Read the model definition and answer for the solid it produces. Units are mm, in the model's axes. Face numbers are marked on the shaded views. A direction names the side the tool comes from. Give positions to 0.01 mm unless a question says otherwise; leave off trailing zeros. Write each loop counter-clockwise with the first axis right and the second up, starting at its lowest first coordinate (ties: lowest second). Pieces come first, ordered by that corner, then holes.
```python
from build123d import *

# Parameters (mm, degrees)
SKETCH1_W           = 19.05
SKETCH1_H           = 57.15
BOSS_EXTRUDE1_DEPTH = 25.4
SKETCH2_W           = 17.4625
SKETCH2_H           = 19.05
SKETCH2_W_2         = 9.525
CUT_EXTRUDE1_DEPTH  = 20.05
SKETCH9_R           = 3.175
CUT_EXTRUDE3_DEPTH  = 40.6875
FILLET1_R           = 6.35
HOLE1_D             = 7.874
CHAMFER1_SIZE       = 0.508


with BuildPart() as part:
    # Sketch1 → Boss-Extrude1 (new body)
    with BuildSketch(Plane(origin=(0, 0, 0), x_dir=(1, 0, 0), z_dir=(0, 1, 0))):
        with Locations((69.85, 0)):
            Rectangle(SKETCH1_W, SKETCH1_H)
    extrude(amount=BOSS_EXTRUDE1_DEPTH)

    # Sketch2 → Cut-Extrude1 (cut, through all)
    with BuildSketch(Plane(origin=(79.375, 0, 0), x_dir=(0, 0, -1), z_dir=(1, 0, 0))):
        with Locations((-19.84375, 15.875)):
            Rectangle(SKETCH2_W, SKETCH2_H)
        with Locations((0, 15.875)):
            Rectangle(SKETCH2_W_2, SKETCH2_H)
        with Locations((19.84375, 15.875)):
            Rectangle(SKETCH2_W, SKETCH2_H)
    extrude(amount=-CUT_EXTRUDE1_DEPTH, mode=Mode.SUBTRACT)

    # Sketch9 → Cut-Extrude3 (cut, through all)
    with BuildSketch(Plane.XY.offset(11.1125)):
        with Locations((69.85, 19.05)):
            Circle(SKETCH9_R)
    extrude(amount=-CUT_EXTRUDE3_DEPTH, mode=Mode.SUBTRACT)

    # Fillet1
    fillet1_edges = [part.edges().sort_by_distance(p)[0] for p in [
        (79.375, 25.4, 7.9375),
        (79.375, 3.175, 28.575),
        (60.325, 3.175, 28.575),
        (79.375, 25.4, -7.9375),
        (60.325, 25.4, -7.9375),
        (60.325, 25.4, 7.9375),
        (60.325, 3.175, -28.575),
        (79.375, 3.175, -28.575),
    ]]
    fillet(fillet1_edges, radius=FILLET1_R)

    # Hole1 (through all)
    with Locations(Plane(origin=(0, 6.35, 0), x_dir=(1, 0, 0), z_dir=(0, 1, 0))):
        with Locations((69.923370565, 18.735910675), (69.923370565, -18.735910675)):
            Hole(HOLE1_D / 2)

    # Chamfer1
    chamfer1_edges = [part.edges().sort_by_distance(p)[0] for p in [
        (73.860370565, 6.35, 18.735910675),
        (73.860370565, 0, 18.735910675),
        (73.860370565, 6.35, -18.735910675),
        (73.860370565, 0, -18.735910675),
    ]]
    chamfer(chamfer1_edges, length=CHAMFER1_SIZE)


solid = part.part
```
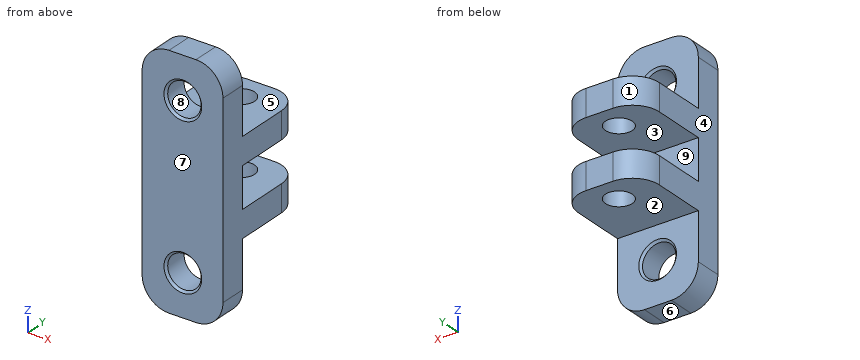
Item 1: Section C-C (y = 21.5) is taken. Write down the section's boundary in (x, z), and give its area (3 significant figures).
Result set:
outline: (60.82, -11.11) - (67.83, -11.11) - (67.83, -4.76) - (60.82, -4.76) - close; (60.82, 4.76) - (67.83, 4.76) - (67.83, 11.11) - (60.82, 11.11) - close; (71.87, -11.11) - (78.88, -11.11) - (78.88, -4.76) - (71.87, -4.76) - close; (71.87, 4.76) - (78.88, 4.76) - (78.88, 11.11) - (71.87, 11.11) - close
area: 178 mm2
Item 2: Section D-D (y = 2.25) is taken. Write down the section's boundary in (x, z) (3 decimals).
Result set:
outline: (60.325, -22.225) arc R6.35 ccw to (66.675, -28.575) - (73.025, -28.575) arc R6.35 ccw to (79.375, -22.225) - (79.375, 22.225) arc R6.35 ccw to (73.025, 28.575) - (66.675, 28.575) arc R6.35 ccw to (60.325, 22.225) - close; hole circle Ø7.874 at (69.923, -18.736); hole circle Ø7.874 at (69.923, 18.736)
Item 3: Determine the mould class of the marked faces 6, 7, 8 and 9 for opening direction Z: pulls with the +Z half, pulls with the -Z half, needs draft (parallel to the pull), parting line crosses it, or undercut.
Result set:
face 6: pulls with the -Z half
face 7: needs draft
face 8: undercut
face 9: undercut
Item 4: Which of the six approach directions +Z, -Z, +X, -X, +Y, -Y give full straight-line access (tool end or side, diameter ignored) to the marked faces 1, 2, 3, 4 and 5?
Result set:
face 1: +Z, -Z, -X, +Y
face 2: -Z, +X, -X, +Y
face 3: +X, -X, +Y
face 4: +Z, -Z, -X, +Y, -Y
face 5: +Z, +X, -X, +Y
Item 5: Each of these flat-tipped pins is pushed along its axis until it touches: pin 1 Ø5 at (x, z) = (73.5, 2.5) entering from +Y; pin 2 Ø10 at (x, y) = (74, 16) entering from +Z; pin 3 Ø5 at (x, z) = (67.5, -23) entering from +Y; pin 4 Ø5.5 at (x, y) = (68, 12) entering from -Z. Where does it stop, or does it pass through?
Result set:
pin 1: stops at y = 25.4
pin 2: stops at z = 11.11
pin 3: stops at y = 6.35
pin 4: stops at z = -11.11
Item 6: Section B-B (z = -7.5) is taken. Write down the section's boundary in (x, y) (3 decimals).
Result set:
outline: (60.325, 0) - (79.375, 0) - (79.375, 19.05) arc R6.35 ccw to (73.025, 25.4) - (66.675, 25.4) arc R6.35 ccw to (60.325, 19.05) - close; hole circle Ø6.35 at (69.85, 19.05)
Item 7: Section A-A (y = 12.5) is taken. Write down the section's boundary in (x, z) (1 decimal).
Result set:
outline: (60.3, -11.1) - (79.4, -11.1) - (79.4, -4.8) - (60.3, -4.8) - close; (60.3, 4.8) - (79.4, 4.8) - (79.4, 11.1) - (60.3, 11.1) - close
Item 8: Find the intervals of material crossed by line 1 along Z through (x, y) = (65.5, 20); line 2 along Z through (x, y) = (67.5, 2) (3 decimals); line 3 along Z through (x, y) = (71.25, 4) (3 decimals), in increasing order.
Result set:
line 1: z = -11.11 to -4.76, 4.76 to 11.11
line 2: z = -28.575 to -21.839, -15.633 to 15.633, 21.839 to 28.575
line 3: z = -28.575 to -22.443, -15.029 to 15.029, 22.443 to 28.575
